Check sheet for the drawn part. Datum: minimum x, y, z corner. Units: mm. A direction names the side the tool comes from. Round coordinates to 2 decimals unless told otherwise and drop trailing zeros. Order: outer loops, then holes, each group sorted by start corner. A loop starts at its lowest first (then second) coordinate and runs counter-clockwise, first axis right, second up.
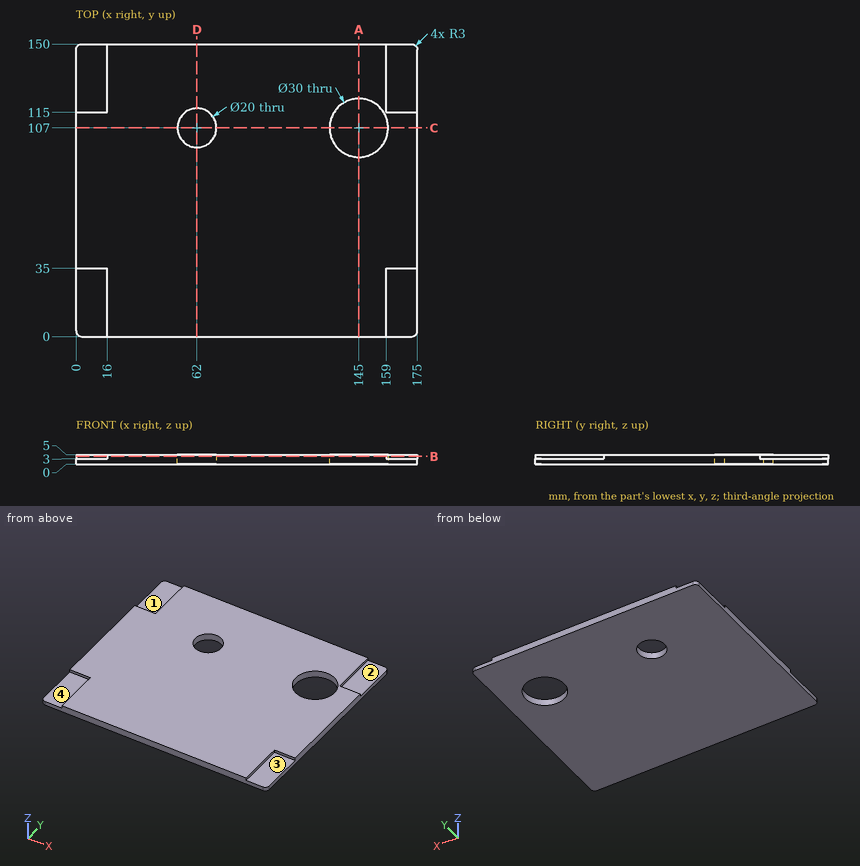
(1) Sectioned sample at A-A, the plane x = 145. Record the cut outline in (y, z), and give its area (3 significant figures).
Returned:
outline: (0, 0) - (92, 0) - (92, 5) - (0, 5) - close; (122, 0) - (150, 0) - (150, 5) - (122, 5) - close
area: 600 mm2
(2) Sectioned sample at C-C, the plane y = 107. Record the cut outline in (x, z), and give its area (3 significant figures).
Returned:
outline: (0, 0) - (52, 0) - (52, 5) - (0, 5) - close; (72, 0) - (130, 0) - (130, 5) - (72, 5) - close; (160, 0) - (175, 0) - (175, 5) - (160, 5) - close
area: 625 mm2
(3) Sectioned sample at D-D, the plane x = 62. Record the cut outline in (y, z), and give its area (3 significant figures).
Returned:
outline: (0, 0) - (97, 0) - (97, 5) - (0, 5) - close; (117, 0) - (150, 0) - (150, 5) - (117, 5) - close
area: 650 mm2
(4) Depth check by flat-ended pin: P1, Ø8, axis at x = 5, y = 138.5, coming from the +Z side; P2, Ø1, axis at x = 6.5, z = 4, coming from the -Y side; P3, Ø2, axis at x = 11, z = 4.5, coming from the +Y side. Enter the tip coordinate at first touch or a pass-through.
Returned:
P1: stops at z = 3
P2: stops at y = 35
P3: stops at y = 115
(5) Set-up check for the marked faces 1, 2, 3 and 4: record each of +Z, -Z, +X, -X, +Y, -Y from which the full face is reachable in a straight line by a thin tool's end or side.
Returned:
face 1: +Z, -X, +Y
face 2: +Z, +X, +Y
face 3: +Z, +X, -Y
face 4: +Z, -X, -Y
(6) Sectioned sample at B-B, the plane z = 4.05. Record the cut outline in (x, y), and give its area (3 significant figures).
Returned:
outline: (0, 35) - (16, 35) - (16, 0) - (159, 0) - (159, 35) - (175, 35) - (175, 115) - (159, 115) - (159, 150) - (16, 150) - (16, 115) - (0, 115) - close; hole circle Ø20 at (62, 107); hole circle Ø30 at (145, 107)
area: 23,000 mm2
(7) Material ranges on line 1 (Y direction, x = 62, z = 2.1); line 2 (Y direction, x = 145, z = 2.45); line 3 (Z direction, x = 12, y = 142.5), recorded low to high.
Returned:
line 1: y = 0 to 97, 117 to 150
line 2: y = 0 to 92, 122 to 150
line 3: z = 0 to 3
